Source: CAD feature listing. Evaluate the final solid. Frame: model axes, mm. Give positions to 0.01 mm unless a question says otherwise; leave off trailing zeros. Order: outer loops, then holes, each group sorted by start corner. A loop starts at its lowest first (then second) coordinate and runs counter-clockwise, first axis right, second up.
Autodesk Inventor part; units mm, degrees
ref_plane "YZ Plane" through (0, 0, 0) normal (1, 0, 0) x (0, 1, 0)
ref_plane "XZ Plane" through (0, 0, 0) normal (0, 1, 0) x (-1, 0, 0)
ref_plane "XY Plane" through (0, 0, 0) normal (0, 0, 1) x (1, 0, 0)
sketch "Esquisse1" plane through (0, 0, 0) normal (0, 1, 0) x (-1, 0, 0)
  line L0 (-11.5, 25) -> (11.5, 25)
  line L1 (12.5, 24) -> (12.5, -24)
  line L2 (11.5, -25) -> (-11.5, -25)
  line L3 (-12.5, -24) -> (-12.5, 24)
  line L4 (-12.5, 25) -> (12.5, -25) construction
  line L5 (12.5, 25) -> (-12.5, -25) construction
  arc A0 (12.5, 24) -> (11.5, 25) centre (11.5, 24) ccw
  arc A1 (-11.5, 25) -> (-12.5, 24) centre (-11.5, 24) ccw
  arc A2 (-12.5, -24) -> (-11.5, -25) centre (-11.5, -24) ccw
  arc A3 (11.5, -25) -> (12.5, -24) centre (11.5, -24) ccw
  line L6 (0, 25) -> (0, 22.5) construction
  circle A4 centre (0, 22.5) radius 1.75
  line L7 (9.4717, 25) -> (9.4717, -7) construction
  line L8 (12.5, -7) -> (10, -7) construction
  circle A5 centre (10, -7) radius 1.75
  circle A6 centre (-10, -7) radius 1.75
  point P0 (0, 0)
  dimension "d0" = 25
  dimension "d1" = 50
  dimension "d2" = 1
  dimension "d3" = 2.5
  dimension "d4" = 3.5
  dimension "d5" = 32
  dimension "d6" = 2.5
  dimension "d7" = 3.5
extrude "Extrusion1" add sketch "Esquisse1" along normal blind 1.5
sketch "Sketch2" plane through (-12.5, 0, -24) normal (-1, 0, 0) x (0, 0, 1)
  point P0 (24, 0)
sketch "Sketch3" plane through (0, 1.5, 0) normal (0, 1, 0) x (1, 0, 0)
  point P0 (0, 0)
properties part number "PCB"
(1) Section C-C, the plane y = 1.1. Return loops of the section in (x, z), plus the area to 3 significant figures.
(2) Draft query along Z for faces 1 (the cylindrical face through (9.19, 0.74, -5.45)), 2 (the cylindrical face through (12.199, 0.74, -24.715)), 3 (the flat face through (-12.5, 1, 0)). Return one class per face: +Z half, -Z half, draft (parallel to the pull), parting line (faces both ways), or undercut.
(3) Section B-B, the plane z = 22.5. Return loops of the section in (x, y), plus the area to 4 significant figures.
(4) Section D-D, the plane z = -7. Return loops of the section in (x, y), plus the area to 3 significant figures.
(5) Line query: line 1 along Z through (x, y) = (10, 0.6); line 2 along Z through (x, y) = (0, 0.9). Output: solid intervals per line, ascending.
(6) Section A-A, the plane x = 10. Return loops of the section in (y, z).
Checks:
1. outline: (-12.5, -24) arc R1 ccw to (-11.5, -25) - (11.5, -25) arc R1 ccw to (12.5, -24) - (12.5, 24) arc R1 ccw to (11.5, 25) - (-11.5, 25) arc R1 ccw to (-12.5, 24) - close; hole circle Ø3.5 at (-10, -7); hole circle Ø3.5 at (0, 22.5); hole circle Ø3.5 at (10, -7)
1. area: 1,220 mm2
2. face 1: undercut
2. face 2: -Z half
2. face 3: draft
3. outline: (-12.5, 0) - (-1.75, 0) - (-1.75, 1.5) - (-12.5, 1.5) - close; (1.75, 0) - (12.5, 0) - (12.5, 1.5) - (1.75, 1.5) - close
3. area: 32.25 mm2
4. outline: (-12.5, 0) - (-11.75, 0) - (-11.75, 1.5) - (-12.5, 1.5) - close; (-8.25, 0) - (8.25, 0) - (8.25, 1.5) - (-8.25, 1.5) - close; (11.75, 0) - (12.5, 0) - (12.5, 1.5) - (11.75, 1.5) - close
4. area: 27.0 mm2
5. line 1: z = -25 to -8.75, -5.25 to 25
5. line 2: z = -25 to 20.75, 24.25 to 25
6. outline: (0, -25) - (1.5, -25) - (1.5, -8.75) - (0, -8.75) - close; (0, -5.25) - (1.5, -5.25) - (1.5, 25) - (0, 25) - close
